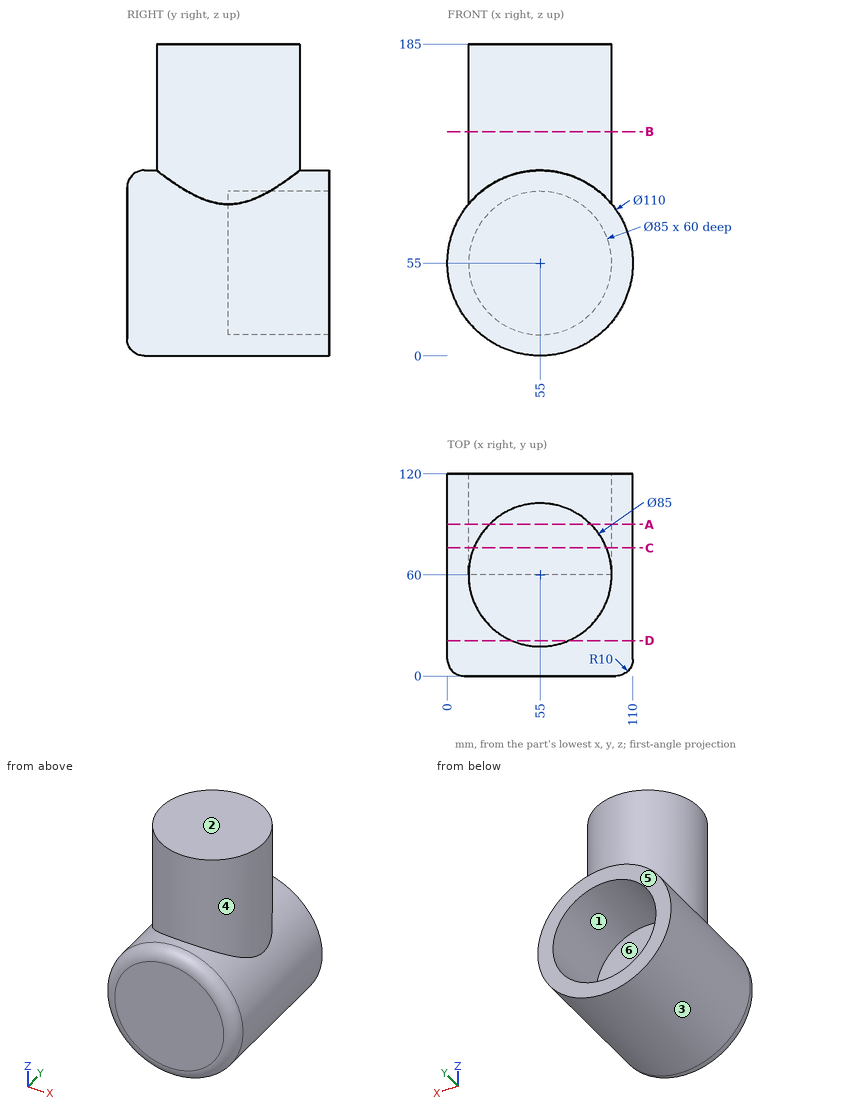
Part print with two shaded views. Sizes in mm from the minimum x, y, z corner. A direction names the side the tool comes from. Round coordinates to 2 decimals unless told otherwise and drop trailing zeros. Loops run counter-clockwise (first coordinate to the right, second up) from the corner with the lowest first, then second, coordinate; pieces in that order, holes last. Notation, with made-up numbers: M 12.5,-18 L 53.5,-18 A32 cw 53.5,20 Z; hole C 86.25,77.5 d10. An arc over 180 degrees is marked long. Return JSON: item names as keys, results as strings. Group by question number.
(1) Tool access for the marked faces 4, 5 and 6: list every direction of +Z, -Z, +X, -X, +Y, -Y with a clear straight run to the whole face (end or side of a thin tool).
(2) Saw through at D-D, the plane y = 21. List the corners of the cut face in (x, z), and give its area (3 significant figures).
(3) Drop flat-ended pins along their axis: P1, Ø1.5, axis at y = 34.5, z = 158.5, coming from the -X side; P2, Ø3, axis at x = 88, y = 76.5, coming from the -Z side; P3, Ø8, axis at x = 50.5, z = 133.5, coming from the +Y side. Give the stop position or say it passes through.
(4) Saw through at C-C, the plane y = 76. List the corners of the cut face in (x, z), and give its area (3 significant figures).
(5) Saw through at A-A, the plane y = 90. List the corners of the cut face in (x, z).
(6) Mould opens along X. For the marked faces 1, 2 and 3 say: +X half, -X half, draft (parallel to the pull), parting line (faces both ways), or undercut.
(7) Wall check: probe 1 along Z at (x, y) = (55, 101); probe 2 along Z at (x, y) = (55, 105); probe 3 along Y at (x, z) = (69.5, 63.5). Give the ranges that are in metal, low to high. Write a range as [from, to].
(8) Saw through at B-B, the plane z = 133. List the corners of the cut face in (x, y), and give its area (3 significant figures).
Answer list:
{
 "1": {"face 4": "+Z", "face 5": "+Z, -Z, +X, -X, +Y", "face 6": "+Y"},
 "2": {"outline": "M 38.11,107.34 A55 ccw long 71.89,107.34 L 71.89,185 L 38.11,185 Z", "area": "12,100 mm2"},
 "3": {"P1": "x = 20.45", "P2": "z = 9.91", "P3": "y = 102.5"},
 "4": {"outline": "M 15.63,93.4 A55 ccw long 94.37,93.4 L 94.37,185 L 15.63,185 Z; hole C 55,55 d85", "area": "10,100 mm2"},
 "5": {"outline": "M 24.9,101.03 A55 ccw long 85.1,101.03 L 85.1,185 L 24.9,185 Z; hole C 55,55 d85"},
 "6": {"face 1": "undercut", "face 2": "draft", "face 3": "parting line"},
 "7": {"probe 1": "[0, 12.5], [97.5, 185]", "probe 2": "[0, 12.5], [97.5, 110]", "probe 3": "[0, 60]"},
 "8": {"outline": "C 55,60 d85", "area": "5,670 mm2"}
}
